from build123d import *

# Parameters (mm, degrees)
F1_DEPTH = 63.5
F2_DEPTH = 25.4
F3_DEPTH = 7.9375


with BuildPart() as f1:
    # F0 (on Front) → F1 (new body, symmetric)
    with BuildSketch(Plane.XZ):
        Polygon((-41.275, -9.525), (41.275, -9.525), (41.275, 9.525), (22.225, 9.525), (-41.275, 9.525), align=None)
    extrude(amount=F1_DEPTH, both=True)

    # F0 (on Front) → F2 (join, symmetric)
    with BuildSketch(Plane.XZ):
        with BuildLine():
            Line((22.225, 9.525), (41.275, 9.525))
            Line((41.275, 9.525), (41.275, 27.0002))
            ThreePointArc((41.275, 27.0002), (45.9246798487, 38.2255201513), (57.15, 42.8752))
            Line((57.15, 42.8752), (60.325, 42.8752))
            Line((60.325, 42.8752), (60.325, 61.9252))
            Line((60.325, 61.9252), (57.15, 61.9252))
            add(Edge.make_bspline(
                [(50.7054314014, 61.3254554335), (52.822029921, 61.5361395895), (54.9703769796, 61.7357484347), (57.15, 61.9252)],
                knots=[107.251905299, 107.251905299, 107.251905299, 107.251905299, 111.5045361635, 111.5045361635, 111.5045361635, 111.5045361635], degree=3))
            ThreePointArc((50.7054314014, 61.3254554335), (30.2722007662, 49.3013105855), (22.225, 27.0002))
            Line((22.225, 27.0002), (22.225, 9.525))
        make_face()
        Polygon((60.325, 61.9252), (60.325, 42.8752), (60.325, 38.1), (85.725, 38.1), (85.6410190463, 66.675), (60.325, 66.675), align=None)
    extrude(amount=F2_DEPTH, both=True)

    # F0 (on Front) → F3 (join, symmetric)
    with BuildSketch(Plane.XZ):
        with BuildLine():
            add(Edge.make_bspline(
                [(-41.275, 9.525), (-35.8625339524, 43.6539850574), (-2.675459444, 56.0119735297), (50.7054314014, 61.3254554335)],
                knots=[0, 0, 0, 0, 107.251905299, 107.251905299, 107.251905299, 107.251905299], degree=3))
            Line((-41.275, 9.525), (22.225, 9.525))
            Line((22.225, 9.525), (22.225, 27.0002))
            ThreePointArc((22.225, 27.0002), (30.2722007662, 49.3013105855), (50.7054314014, 61.3254554335))
        make_face()
    extrude(amount=F3_DEPTH, both=True)

    # F0 (on Front) → F4 (revolve)
    with BuildSketch(Plane.XZ):
        Polygon((85.6410190463, 66.675), (85.725, 38.1), (111.125, 38.1), (111.125, 66.675), align=None)
    revolve(axis=Axis((85.6830095232, 0, 52.3875), (-0.0029389533, 0, 0.9999956813)))


solid = f1.part
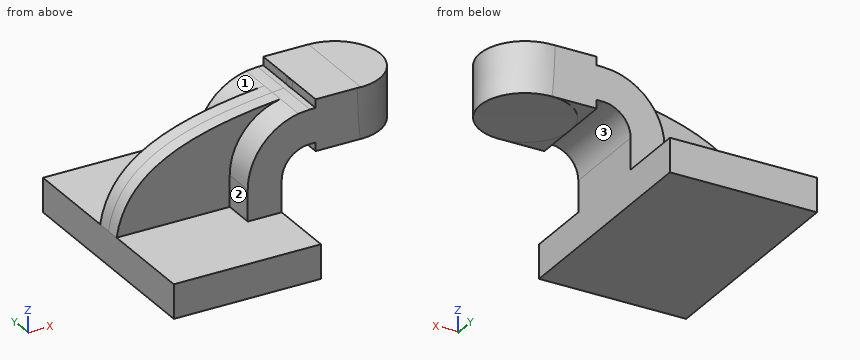
Geometry check sheet. Reference: the model listing, model coordinates, mm. Face numbers are marked on the shaded views. A direction names the side the tool comes from. Give positions to 0.01 mm unless a question says otherwise; leave off trailing zeros. Loops run counter-clockwise (first coordinate to the right, second up) from the corner with the lowest first, then second, coordinate; pieces in that order, holes last.
(1) Depth check by flat-ended pin: pin 1 Ø1 at (x, y) = (59, -10) entering from +Z; pin 2 Ø1 at (y, z) = (11, 12) entering from -X (3 decimals); pin 3 Ø2.5 at (y, z) = (7, 39.5) entering from -X. Enter the tip coordinate at first touch or a pass-through.
From the geometry:
pin 1: stops at z = 61.93
pin 2: stops at x = 22.225
pin 3: stops at x = -25.41
(2) Section check A-A on z = 0.5. Record the cut outline in (x, y) (3 decimals).
From the geometry:
outline: (-41.275, -63.5) - (41.275, -63.5) - (41.275, 63.5) - (-41.275, 63.5) - close
(3) Set-up check for the marked faces 1, 2 and 3: record each of +Z, -Z, +X, -X, +Y, -Y from which the full face is reachable in a straight line by a thin tool's end or side.
From the geometry:
face 1: +Z, -X, +Y
face 2: +Z, -X, -Y
face 3: -Z, +Y, -Y
(4) Thickness scan on L1, parallel to Z at x = 28, y = -27 (3 decimals); L2, parallel to Y at x = -3.5, z = 45; L3, parallel to Y at x = 81, z = 39. Record the ranges inside material, lowest first.
From the geometry:
L1: z = -9.525 to 9.525
L2: y = -7.94 to 7.94
L3: y = -25.4 to 25.4
(5) Section check B-B on y = -52.5. Record the cut outline in (x, z) (3 decimals), then the cut area to 3 significant figures.
From the geometry:
outline: (-41.275, -9.525) - (41.275, -9.525) - (41.275, 9.525) - (-41.275, 9.525) - close
area: 1,570 mm2
